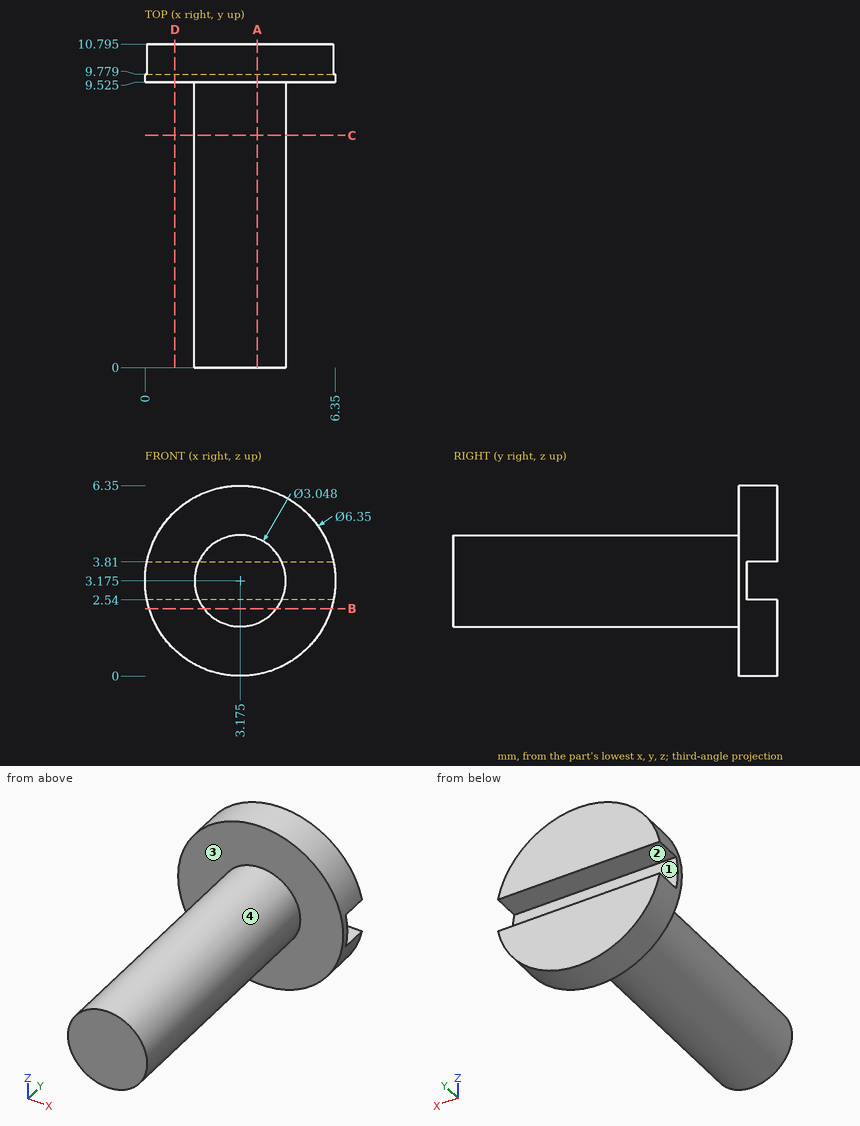
Part print with two shaded views. Sizes in mm from the minimum x, y, z corner. Round coordinates to 2 decimals unless told otherwise and drop trailing zeros. Loops run counter-clockwise (first coordinate to the right, second up) from the corner with the lowest first, then second, coordinate; pieces in that order, holes last.
Item 1: Two-plate mould, pull along Z, no slides. Class the marked faces 1, 2, 3 and 4: released by +Z, released by -Z, zero draft, split by the parting line, or undercut.
Item 2: Pin check, flat tips, straight feed: P1, Ø0.5, axis at x = 2.5, y = 10.5, coming from the +Z side; P2, Ø2, axis at x = 2.5, y = 7.5, coming from the -Z side. Stop position of each tip, or through.
Item 3: Saw through at B-B (z = 2.25). List the corners of the cut face in (x, y) (3 decimals).
Item 4: Drill centre lines: line 1 along Z through (x, y) = (3.25, 0.75); line 2 along Y through (x, z) = (0.75, 4.75) (3 decimals); line 3 along Z through (x, y) = (3.5, 10.25). Where is each one in solid material? Low to high.
Item 5: Saw through at C-C (y = 7.75). List the corners of the cut face in (x, z) (3 decimals).
Item 6: Saw through at D-D (x = 1). List the corners of the cut face in (y, z) (3 decimals), then the cut area to 3 significant figures.
Item 7: Saw through at A-A (x = 3.75). List the corners of the cut face in (y, z) (1 decimal).
Worked answers:
1. face 1: undercut
1. face 2: undercut
1. face 3: zero draft
1. face 4: split by the parting line
2. P1: stops at z = 6.32
2. P2: stops at z = 1.65
3. outline: (0.138, 9.525) - (1.964, 9.525) - (1.964, 0) - (4.386, 0) - (4.386, 9.525) - (6.212, 9.525) - (6.212, 10.795) - (0.138, 10.795) - close
4. line 1: z = 1.65 to 4.7
4. line 2: y = 9.525 to 10.795
4. line 3: z = 0.02 to 2.54, 3.81 to 6.33
5. outline: circle Ø3.048 at (3.175, 3.175)
6. outline: (9.525, 0.862) - (10.795, 0.862) - (10.795, 2.54) - (9.779, 2.54) - (9.779, 3.81) - (10.795, 3.81) - (10.795, 5.488) - (9.525, 5.488) - close
6. area: 4.58 mm2
7. outline: (0, 1.8) - (9.5, 1.8) - (9.5, 0.1) - (10.8, 0.1) - (10.8, 2.5) - (9.8, 2.5) - (9.8, 3.8) - (10.8, 3.8) - (10.8, 6.3) - (9.5, 6.3) - (9.5, 4.6) - (0, 4.6) - close
